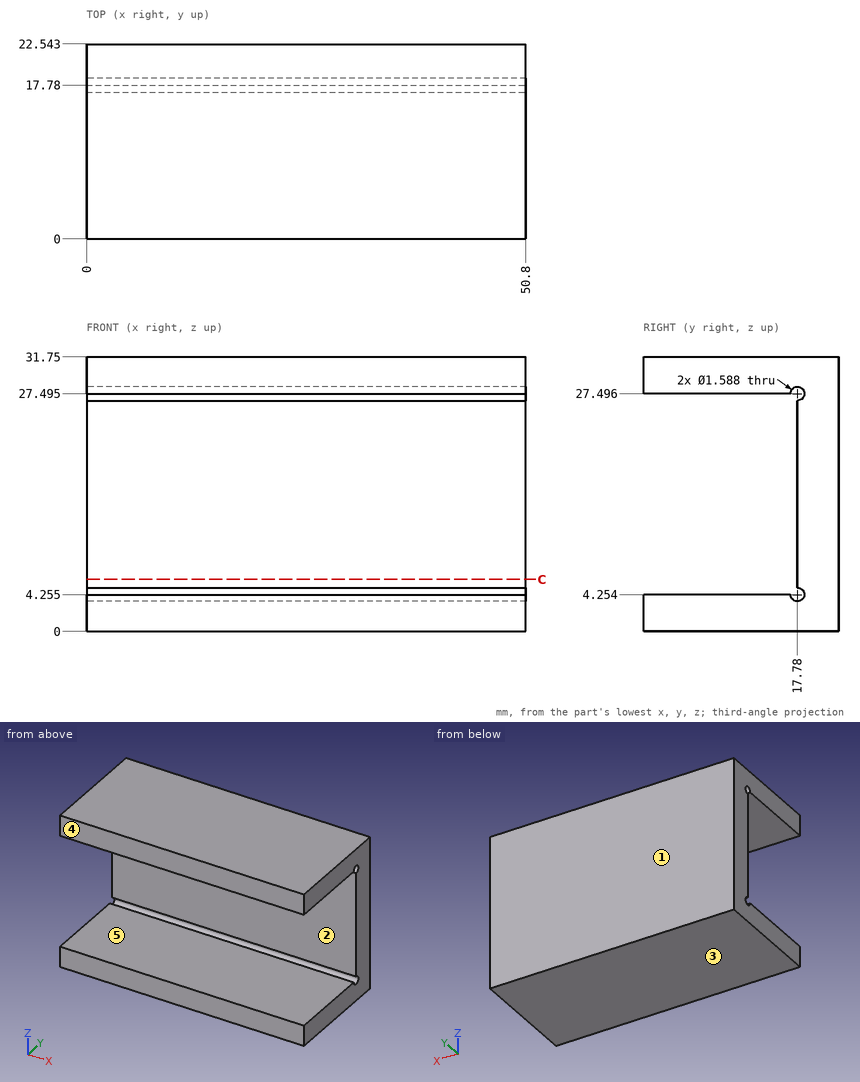
Study the drawing (mm; zero at the part's minimum x, y, z) and answer. A direction names the side the tool comes from. Give positions to 0.01 mm unless a question says otherwise; leave off trailing zeros. Loops run counter-clockwise (first coordinate to the right, second up) from the corner with the lowest first, then second, coordinate; pieces in that order, holes last. Notation, with made-up numbers: M 18,81.5 L 42,81.5 A28 ccw 42,110.5 Z; hole C 21.5,26.5 d6. An arc over 180 degrees is marked long. One line per item, written item: value. Start each with the question number.
1. Determine the mould class of the marked faces 1, 2 and 3 for opening direction Z: released by +Z, released by -Z, zero draft, split by the parting line, or undercut.
2. Find section C-C (z = 6). Give the vertices of the cut face in (x, y), and give its area (3 significant figures).
3. Each of these flat-tipped pins is pushed along its axis until it touches: P1, Ø5, axis at x = 23, z = 18, coming from the -Y side; P2, Ø1.3, axis at y = 17.78, z = 4.25, coming from the -X side. Where does it stop, or does it pass through?
4. Which of the six approach directions +Z, -Z, +X, -X, +Y, -Y give full straight-line access (tool end or side, diameter ignored) to the marked faces 4 and 5?
5. Find the intervals of material crossed by probe 1 along Y at (x, z) = (25.5, 10); probe 2 along Y at (x, z) = (26, 4); probe 3 along Z at (x, y) = (41, 17.5), in increasing order.
Reported:
1. face 1: zero draft
1. face 2: undercut
1. face 3: released by -Z
2. outline: M 0,17.78 L 50.8,17.78 L 50.8,22.54 L 0,22.54 Z
2. area: 242 mm²
3. P1: stops at y = 17.78
3. P2: passes through
4. face 4: +Z, -Z, +X, -X, -Y
4. face 5: +X, -X, -Y
5. probe 1: y = 17.78 to 22.54
5. probe 2: y = 0 to 17.03, 18.53 to 22.54
5. probe 3: z = 0 to 3.51, 28.24 to 31.75
